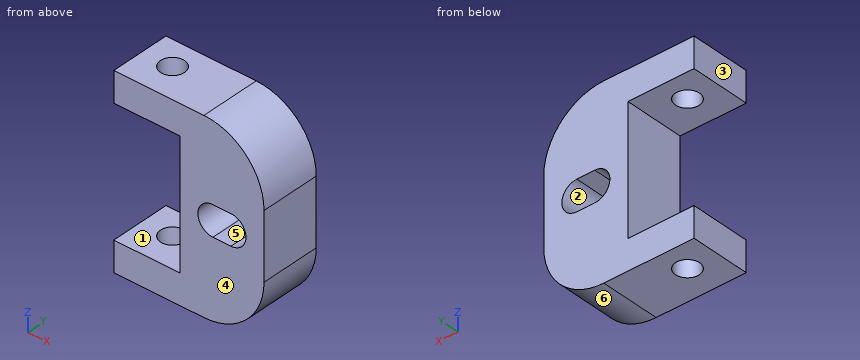
```python
from build123d import *

# Parameters (mm, degrees)
F0_W      = 25
F0_H      = 10
F1_DEPTH  = 15.5
F2_W      = 11
F2_H      = 21
F3_DEPTH  = 10.001
F4_R      = 2.5
F5_DEPTH  = 10.001
F6_R      = 10
F7_R      = 2
F8_DEPTH  = 16
F10_DEPTH = 25


with BuildPart() as f1:
    # F0 (on Top) → F1 (new body, symmetric)
    with BuildSketch(Plane.XY):
        with Locations((12.5, 5)):
            Rectangle(F0_W, F0_H)
    extrude(amount=F1_DEPTH, both=True)

    # F2 (on face) → F3 (cut, through all)
    with BuildSketch(Plane(origin=(0, 10, 0), x_dir=(-1, 0, 0), z_dir=(0, 1, 0))):
        with Locations((-5.5, 0)):
            Rectangle(F2_W, F2_H)
    extrude(amount=-F3_DEPTH, mode=Mode.SUBTRACT)

    # F4 (on face) → F5 (cut, through all)
    with BuildSketch(Plane(origin=(0, 10, 0), x_dir=(-1, 0, 0), z_dir=(0, 1, 0))):
        with Locations((-18, 0)):
            Circle(F4_R)
    extrude(amount=-F5_DEPTH, mode=Mode.SUBTRACT)

    # F6
    f6_edges = [f1.edges().sort_by_distance(p)[0] for p in [
        (25, 5, -15.5),
        (25, 5, 15.5),
    ]]
    fillet(f6_edges, radius=F6_R)

    # F7 (on Top) → F8 (cut, symmetric)
    with BuildSketch(Plane.XY):
        with Locations((5, 5.5)):
            Circle(F7_R)
    extrude(amount=F8_DEPTH, both=True, mode=Mode.SUBTRACT)

    # F9 (on face) → F10 (cut)
    with BuildSketch(Plane.XZ):
        with BuildLine():
            Line((19.5, 2.5), (16.5, 2.5))
            ThreePointArc((16.5, 2.5), (14, 0), (16.5, -2.5))
            Line((16.5, -2.5), (19.5, -2.5))
            ThreePointArc((19.5, -2.5), (22, 0), (19.5, 2.5))
        make_face()
    extrude(amount=-F10_DEPTH, mode=Mode.SUBTRACT)


solid = f1.part
```
For this review, take the finished solid that the model builds, in its own axes (mm). Face numbers are marked on the shaded views. A direction names the side the tool comes from. Give positions to 0.01 mm unless a question says otherwise; leave off trailing zeros. Write each loop counter-clockwise with the first axis right and the second up, starting at its lowest first coordinate (ties: lowest second). Pieces come first, ordered by that corner, then holes.
Item 1: Take a section at D-D (y = 8.75). Give the boundary of the cut face in (x, z).
Item 2: Insertion check: P1, Ø0.9, axis at x = 17.5, y = 5.5, coming from the -Z side; P2, Ø3, axis at y = 7.5, z = 2.5, coming from the -X side; P3, Ø0.9, axis at x = 18, y = 4, coming from the +Z side. Each pin has a flat end and moves straight along its axis. Give the tip position at first contact, or say it passes through.
Item 3: Take a section at C-C (x = 5). Give the boundary of the cut face in (y, z).
Item 4: Take a section at B-B (z = 0). Give the boundary of the cut face in (x, y).
Item 5: Take a section at A-A (y = 5.5). Give the boundary of the cut face in (x, z), and give its area (3 significant figures).
Item 6: The part is to be moulded in two halves that separate along Z. For the marked faces 4, 5 and 6, say which applies: +Z half, -Z half, draft (parallel to the pull), parting line (faces both ways), or undercut.
Item 7: Wall thickness on probe 1 along Z at (x, y) = (9.5, 5.5); probe 2 along Y at (x, z) = (5, -13.6); probe 3 along X at (y, z) = (1.25, -2): over which ranges is each line inside the solid? List them lowest first.
Item 8: Machinability: for the marked faces 1, 2 and 3, which of the approach directions +Z, -Z, +X, -X, +Y, -Y give a long, thin tool a straight path to every point of the face, cutting with its end or side? Answer none if there is none.
Established:
1. outline: (0, -15.5) - (15, -15.5) arc R10 ccw to (25, -5.5) - (25, 5.5) arc R10 ccw to (15, 15.5) - (0, 15.5) - (0, 10.5) - (11, 10.5) - (11, -10.5) - (0, -10.5) - close; hole (16.5, -2.5) - (19.5, -2.5) arc R2.5 ccw to (19.5, 2.5) - (16.5, 2.5) arc R2.5 ccw to start
2. P1: stops at z = -15.29
2. P2: stops at x = 11
2. P3: stops at z = 15.17
3. outline: (0, -15.5) - (3.5, -15.5) - (3.5, -10.5) - (0, -10.5) - close; (0, 10.5) - (3.5, 10.5) - (3.5, 15.5) - (0, 15.5) - close; (7.5, -15.5) - (10, -15.5) - (10, -10.5) - (7.5, -10.5) - close; (7.5, 10.5) - (10, 10.5) - (10, 15.5) - (7.5, 15.5) - close
4. outline: (11, 0) - (14, 0) - (14, 10) - (11, 10) - close; (22, 0) - (25, 0) - (25, 10) - (22, 10) - close
5. outline: (0, -15.5) - (3, -15.5) - (3, -10.5) - (0, -10.5) - close; (0, 10.5) - (3, 10.5) - (3, 15.5) - (0, 15.5) - close; (7, -15.5) - (15, -15.5) arc R10 ccw to (25, -5.5) - (25, 5.5) arc R10 ccw to (15, 15.5) - (7, 15.5) - (7, 10.5) - (11, 10.5) - (11, -10.5) - (7, -10.5) - close; hole (16.5, -2.5) - (19.5, -2.5) arc R2.5 ccw to (19.5, 2.5) - (16.5, 2.5) arc R2.5 ccw to start
5. area: 426 mm2
6. face 4: draft
6. face 5: undercut
6. face 6: -Z half
7. probe 1: z = -15.5 to -10.5, 10.5 to 15.5
7. probe 2: y = 0 to 3.5, 7.5 to 10
7. probe 3: x = 11 to 15, 21 to 25
8. face 1: -X, +Y, -Y
8. face 2: +Y, -Y
8. face 3: +Z, -Z, -X, +Y, -Y
